Could you check a few things on this drawing? It's one solid part, dimensions in mm from its lowest x, y, z. A direction names the side the tool comes from. Give positions to 0.01 mm unless a question says otherwise; leave off trailing zeros. Loops run counter-clockwise (first coordinate to the right, second up) from the corner with the lowest first, then second, coordinate; pieces in that order, holes last.
Q1. Suppose I cut it at B-B (x = 33.5). List the corners of the cut face in (y, z) for me, and give its area (3 significant figures).
Q2. Suppose I cut it at A-A (z = 32). List the corners of the cut face in (x, y) for me (1 decimal).
Q3. Suppose I cut it at C-C (y = 67.5). List the corners of the cut face in (x, z) for me (1 decimal), and give its area (3 significant figures).
Q4. I need wall thicknesses on probe 1 along Y at (x, z) = (15.5, 12.5); probe 2 along X at (y, z) = (78, 29) (1 decimal); probe 3 along Z at (x, y) = (43, 30). Which ranges of each line are inside material? Lowest first, please.
Q5. I'm going to push flat-ended pins straight in: P1, Ø18, axis at y = 33.5, z = 23, coming from the +X side (3 decimals); P2, Ø8, axis at y = 42.5, z = 24, coming from the -X side; P3, Ø13.5, axis at x = 37.5, y = 34.5, coming from the -Z side. Where does each tip first touch, or does it pass through?
Q6. For the marked faces 1, 2, 3 and 4, which set-ups out of +Z, -Z, +X, -X, +Y, -Y let a thin tool reach every point of the face, with its end or its side?
Q7. Suppose I cut it at D-D (z = 6.5). List the corners of the cut face in (x, y) for me, and give its area (4 significant figures).
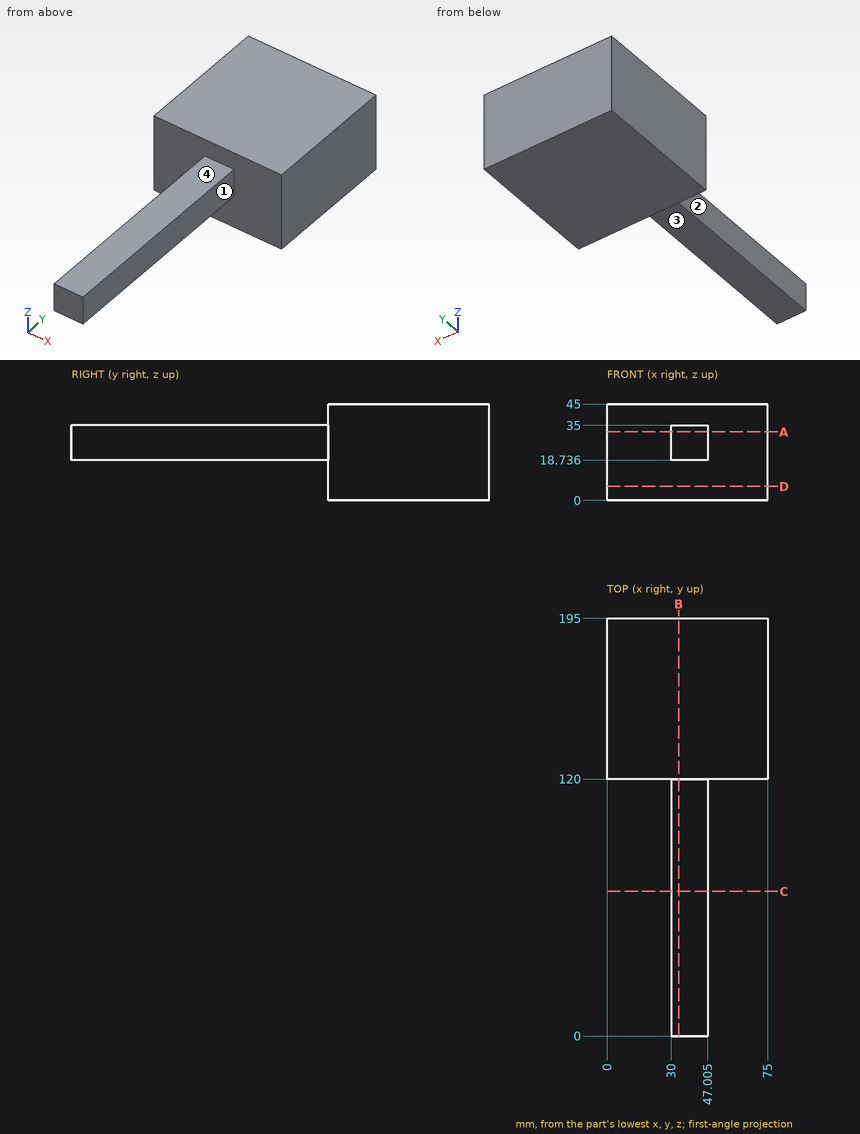
Solutions:
1. outline: (0, 18.74) - (120, 18.74) - (120, 0) - (195, 0) - (195, 45) - (120, 45) - (120, 35) - (0, 35) - close
1. area: 5,330 mm2
2. outline: (0, 120) - (30, 120) - (30, 0) - (47, 0) - (47, 120) - (75, 120) - (75, 195) - (0, 195) - close
3. outline: (30, 18.7) - (47, 18.7) - (47, 35) - (30, 35) - close
3. area: 277 mm2
4. probe 1: y = 120 to 195
4. probe 2: x = 30 to 47
4. probe 3: z = 18.74 to 35
5. P1: stops at x = 47.005
5. P2: stops at x = 30
5. P3: stops at z = 18.74
6. face 1: +Z, -Z, +X, -Y
6. face 2: +Z, -Z, -X, -Y
6. face 3: -Z, +X, -X, -Y
6. face 4: +Z, +X, -X, -Y
7. outline: (0, 120) - (75, 120) - (75, 195) - (0, 195) - close
7. area: 5,625 mm2
